Source: CAD feature listing. Evaluate the final solid. Frame: model axes, mm. A direction names the side the tool comes from. Give positions to 0.01 mm unless a question says otherwise; leave off trailing zeros. Order: outer loops, then holes, each group sorted by start corner. A loop starts at its lowest first (then second) coordinate and runs counter-clockwise, first axis right, second up. Notation, with made-up numbers: M 79,24.25 L 118,24.25 A31 cw 118,51.25 Z; hole C 71,5.5 d10. An arc over 180 degrees is marked long. Return JSON: item names as keys, results as strings.
from build123d import *

# Parameters (mm, degrees)
SKETCH_1_R          = 3.25
EXTRUDE_1_DEPTH     = 28
SKETCH_3_R          = 4.25
CUT_EXTRUDE_1_DEPTH = 17


with BuildPart() as part:
    # 草图1 → 凸台-拉伸1 (new, symmetric)
    with BuildSketch(Plane.XY):
        with BuildLine():
            Line((-77.585786438, 0), (0, 0))
            Line((0, 0), (0, 8))
            Line((0, 8), (-17.995464086, 8))
            Line((-17.995464086, 8), (-30.499317942, 38.186973559))
            Line((-30.499317942, 38.186973559), (-17.774603256, 50.911688245))
            Line((-17.774603256, 50.911688245), (-23.431457505, 56.568542495))
            Line((-23.431457505, 56.568542495), (-78.292893219, 1.707106781))
            ThreePointArc((-78.292893219, 1.707106781), (-78.50966597, 0.617316568), (-77.585786438, 0))
        make_face()
        with Locations((-57.82689122, 9.184402377)):
            Circle(SKETCH_1_R, mode=Mode.SUBTRACT)
        Polygon((-67.928932188, 5), (-63.07447047, 5), (-64.496309389, 8.4326228), align=None, mode=Mode.SUBTRACT)
        with BuildLine():
            Line((-54.257468753, 5), (-20, 5))
            Line((-20, 5), (-34.038059223, 38.890872965))
            Line((-34.038059223, 38.890872965), (-58.261747684, 14.667184504))
            ThreePointArc((-58.261747684, 14.667184504), (-52.745553791, 11.289161255), (-54.257468753, 5))
        make_face(mode=Mode.SUBTRACT)
    extrude(amount=EXTRUDE_1_DEPTH, both=True)

    # 草图3 → 切除-拉伸1 (cut)
    with BuildSketch(Plane(origin=(0, 8, 0), x_dir=(1, 0, 0), z_dir=(0, 1, 0))):
        with Locations(Location((-10, 0, 0), (0, 0, 180))):
            Circle(SKETCH_3_R)
    cut_extrude_1 = extrude(amount=-CUT_EXTRUDE_1_DEPTH, mode=Mode.SUBTRACT)

    # 镜向1: 切除-拉伸1 across plane
    add(cut_extrude_1.mirror(Plane(origin=(-11.715728753, 28.284271247, 0), x_dir=(0, 0, 1), z_dir=(-0.3826834323650881, 0.9238795325112875, 0))), mode=Mode.SUBTRACT)


solid = part.part
1. First-contact query: pin 1 (12 mm diameter, centred on x = -23.5, z = -5.5, fed in from +Y); pin 2 (5 mm diameter, centred on x = -57.83, y = 9.18, fed in from -Z); pin 3 (17 mm diameter, centred on x = -38, z = 4.5, fed in from +Y); pin 4 (14.5 mm diameter, centred on x = -6.5, z = 8.5, fed in from +Y). Flat tips, straight axial feed; report the tip coordinate or a pass-through.
Evaluation:
{"pin 1": "stops at y = 56.57", "pin 2": "passes through", "pin 3": "stops at y = 50.5", "pin 4": "stops at y = 8"}
2. Section query B-B (y = 7). Return loops of the section in (x, z).
Evaluation:
{"outline": "M -73,-28 L -65.93,-28 L -65.93,28 L -73,28 Z; M -63.9,-28 L -60.23,-28 L -60.23,28 L -63.9,28 Z; M -55.42,-28 L -52.78,-28 L -52.78,28 L -55.42,28 Z; M -20.83,-28 L 0,-28 L 0,28 L -20.83,28 Z; hole C -10,0 d8.5"}
3. Section query A-A (z = -1). Return loops of the section in (x, y).
Evaluation:
{"outline": "M -78.29,1.71 A1 ccw -77.59,0 L -14.13,0 L -14.13,8 L -18,8 L -30.5,38.19 L -27.77,40.92 L -33.42,46.58 Z; M -27.58,52.42 L -21.92,46.76 L -17.77,50.91 L -23.43,56.57 Z; M -5.87,0 L 0,0 L 0,8 L -5.87,8 Z; hole M -67.93,5 L -63.07,5 L -64.5,8.43 Z; hole C -57.83,9.18 d6.5; hole M -58.26,14.67 A5.5 cw -54.26,5 L -20,5 L -34.04,38.89 Z"}
4. Section query C-C (x = -10). Return loops of the section in (y, z).
Evaluation:
{"outline": "M 0,-28 L 8,-28 L 8,-4.25 L 0,-4.25 Z; M 0,4.25 L 8,4.25 L 8,28 L 0,28 Z"}
5. Set-up query: faces 4 (the face through (-51.1, 22.1, -28)), 5 (the face through (-21.398, 47.288, 0.392)), 6 (the face through (-26.92, 21.71, 0.39)). Return all of +Z, -Z, +X, -X, +Y, -Y with unobstructed straight access to the full face (end or side cutting, diameter ignored); none if empty.
Evaluation:
{"face 4": "-Z, +X, -X, +Y, -Y", "face 5": "+Z, -Z, +X", "face 6": "+Z, -Z"}
6. Draft query along Y for faces 1 (the face through (-20.563, 53.701, 0.392)), 2 (the face through (0, 4, 0)), 3 (the face through (-24.16, 22.88, 0.39)). Return one class per face: pulls with the +Y half, pulls with the -Y half, needs draft (parallel to the pull), parting line crosses it, or undercut.
Evaluation:
{"face 1": "pulls with the +Y half", "face 2": "needs draft", "face 3": "undercut"}
7. Ray query, probe 1 along Y at (x, z) = (-27.5, -21); probe 2 along Z at (x, y) = (-10, 6); probe 3 along Y at (x, z) = (-5.5, -11.5). Return the intervals inside material, ascending.
Evaluation:
{"probe 1": "y = 0 to 5, 23.11 to 30.95, 41.19 to 52.5", "probe 2": "z = -28 to -4.25, 4.25 to 28", "probe 3": "y = 0 to 8"}
8. Section query D-D (y = 31). Return loops of the section in (x, z), then the cut area to 3 significant figures.
Evaluation:
{"outline": "M -49,-28 L -41.93,-28 L -41.93,28 L -49,28 Z; M -30.77,-28 L -27.52,-28 L -27.52,28 L -30.77,28 Z", "area": "578 mm^2"}
